Geometry: final body of the model. Coordinates: model frame, mm. A direction names the side the tool comes from. Coordinates: 2 decimals unless noted, no trailing zeros. Order: outer loops, then holes, each group sorted by start corner. A loop starts at its lowest first (then second) coordinate and runs counter-clockwise, first axis right, second up. Notation, with made-up numbers: M 41.25,53 L 98.25,53 A8 cw 98.25,64 Z; hole C 16.25,61 d8. An arc over 180 degrees is marked long. One line per question, with ' | ' between items.
Autodesk Fusion 360 part; units mm, degrees
sketch "Esboço1" plane through (0, 0, 0) normal (0, 0, 1) x (1, 0, 0) in component "VibePad Gaming"
  line L0 (0, 0) -> (62.9, 0)
  line L1 (62.9, 0) -> (62.9, 39.1)
  line L2 (62.9, 39.1) -> (0, 39.1)
  line L3 (0, 39.1) -> (0, 0)
  line L4 (-10.5, -10.5) -> (72.4, -10.5)
  line L5 (72.4, -10.5) -> (72.4, 48.6)
  line L6 (72.4, 48.6) -> (-10.5, 48.6)
  line L7 (-10.5, 48.6) -> (-10.5, -10.5)
  circle A0 centre (-5.5, 43.6) radius 1.7
  circle A1 centre (67.4, 43.6) radius 1.7
  circle A2 centre (67.4, -5.5) radius 1.7
  circle A3 centre (-5.5, -5.5) radius 1.7
  circle A4 centre (67.4, -5.5) radius 3
  circle A5 centre (67.4, 43.6) radius 3
  circle A6 centre (-5.5, 43.6) radius 3
  circle A7 centre (-5.5, -5.5) radius 3
  dimension "d1" = 62.9
  dimension "d2" = 39.1
  dimension "d3" = 82.9
  dimension "d4" = 59.1
  dimension "d5" = 9.5
  dimension "d6" = 9.5
  dimension "d7" = 3.4
  dimension "d8" = 3.4
  dimension "d9" = 3.4
  dimension "d10" = 3.4
  dimension "d11" = 5
  dimension "d12" = 5
  dimension "d13" = 5
  dimension "d14" = 5
  dimension "d15" = 5
  dimension "d16" = 5
  dimension "d17" = 5
  dimension "d18" = 5
  dimension "d19" = 6
  dimension "d20" = 6
  dimension "d21" = 6
  dimension "d22" = 6
extrude "Extrusão1" add sketch "Esboço1" along normal blind 9.9 from surface at 3.1 contours A4 | A5 | A6 | A7 makes body 1 at (66.0314, 40.9304, 6.4) makes body 2 at (-2.5037, 43.4505, 9.7) makes body 3 at (66.0314, -8.1696, 6.4) makes body 4 at (-2.5037, -5.6495, 9.7) in component "VibePad Gaming"
extrude "Extrusão2" add sketch "Esboço1" along normal blind 13 contours L4 L5 L6 L7 bodies 1 2 3 4 in component "VibePad Gaming"
extrude "Extrusão3" add sketch "Esboço1" along normal blind 3 contours L0 L1 L2 L3 bodies 1 in component "VibePad Gaming"
sketch "Esboço2" plane through (0, 0, 13) normal (0, 0, 1) x (-1, 0, 0) in component "VibePad Gaming"
  circle A0 centre (-67.4, -43.6) radius 1.7
  circle A1 centre (5.5, 5.5) radius 1.7
  line L0 (0, 0) -> (0, -39.1)
  line L1 (0, -39.1) -> (-62.9, -39.1)
  line L2 (-62.9, -39.1) -> (-62.9, 0)
  line L3 (-62.9, 0) -> (0, 0)
  line L4 (10.5, -48.6) -> (10.5, 10.5)
  line L5 (10.5, 10.5) -> (-72.4, 10.5)
  line L6 (-72.4, 10.5) -> (-72.4, -48.6)
  line L7 (-72.4, -48.6) -> (10.5, -48.6)
  circle A2 centre (5.5, -43.6) radius 1.7
  circle A3 centre (-67.4, 5.5) radius 1.7
  line L8 (-20.95, 0) -> (-2.45, 0)
  line L9 (-2.45, 0) -> (-2.45, 10.5)
  line L10 (-2.45, 10.5) -> (-20.95, 10.5)
  line L11 (-20.95, 10.5) -> (-20.95, 0)
  line L12 (10.5, -48.6) -> (10.5, 10.5)
  dimension "d30" = 18.5
  dimension "d31" = 12.95
extrude "Extrusão4" cut sketch "Esboço2" against normal blind 7.5 contours L3 L5 L8 L9 L10 L11 bodies 1 in component "VibePad Gaming"
fillet "Arredondamento1" radius 5 1 edges at (-10.5, 48.6, 6.5) on bodies 1 in component "VibePad Gaming"
fillet "Arredondamento2" radius 5 1 edges at (-10.5, -10.5, 6.5) on bodies 1 in component "VibePad Gaming"
fillet "Arredondamento3" radius 5 2 edges at (72.4, 48.6, 6.5) (72.4, -10.5, 6.5) on bodies 1 in component "VibePad Gaming"
component "VibePad Gaming" placed x (1, 0, 0) y (0, 1, 0) z (0, 0, 1) at (0, 0, 0)
1. Material intervals for line 1 (Y direction, x = -5.5, z = 9.5); line 2 (Y direction, x = 67.4, z = 2.05); line 3 (Y direction, x = 26, z = 7.5), sorted ascending. Write a range as [from, to].
Response values:
line 1: y = [-10.5, -7.2], [-3.8, 41.9], [45.3, 48.6] | line 2: y = [-10.5, -8.5], [-2.5, 40.6], [46.6, 48.6] | line 3: y = [-10.5, 0], [39.1, 48.6]
2. Section C-C, the plane y = 30.5. Output: boundary loops of the cut face in (x, z).
Response values:
outline: M -10.5,0 L 72.4,0 L 72.4,13 L 62.9,13 L 62.9,3 L 0,3 L 0,13 L -10.5,13 Z
3. Section B-B, the plane x = 17. Output: boundary loops of the cut face in (y, z).
Response values:
outline: M -10.5,0 L 48.6,0 L 48.6,13 L 39.1,13 L 39.1,3 L 0,3 L 0,5.5 L -10.5,5.5 Z
4. Section A-A, the plane z = 4.25. Output: boundary loops of the cut face in (x, y).
Response values:
outline: M -10.5,-5.5 A5 ccw -5.5,-10.5 L 67.4,-10.5 A5 ccw 72.4,-5.5 L 72.4,43.6 A5 ccw 67.4,48.6 L -5.5,48.6 A5 ccw -10.5,43.6 Z; hole C -5.5,-5.5 d3.4; hole C -5.5,43.6 d3.4; hole M 0,0 L 62.9,0 L 62.9,39.1 L 0,39.1 Z; hole C 67.4,-5.5 d3.4; hole C 67.4,43.6 d3.4
5. Draft query along X for faces 1 (the face through (30, -10.5, 6)), 2 (the face through (12, -5, 5.5)), 3 (the face through (-10.5, 19, 6)). Return one class per face: pulls with the +X half, pulls with the -X half, needs draft (parallel to the pull), parting line crosses it, or undercut.
Response values:
face 1: needs draft | face 2: undercut | face 3: pulls with the -X half
6. Access query for faces 4 (the face through (70.97, 47.1, 6.59)), 5 (the face through (65, -3.7, 1.5)), 6 (the face through (32, 39.1, 8)). Directions: +Z, -Z, +X, -X, +Y, -Y. A direction counts if a zero-diameter tool reaches every point of the face in a straight line with its end or side. Return the directions, or none.
Response values:
face 4: +Z, -Z, +X, +Y | face 5: -Z | face 6: +Z
7. Pin query (flat end, axial travel): P1, Ø2.5, axis at x = 67.4, y = 43.6, coming from the -Z side; P2, Ø1.5, axis at x = 58, y = 35, coming from the +Z side; P3, Ø2, axis at y = -7, z = 9, coming from the -X side. Return the tip coordinate at first contact, or that it passes through.
Response values:
P1: passes through | P2: stops at z = 3 | P3: stops at x = -10.47
